The figure shows three views and two pictorial views of one solid part (mm, origin at its lowest corner). Answer the questions. Coordinates: 2 decimals unless noted, no trailing zeros. Write each loop counter-clockwise with the first axis right and the second up, starting at its lowest first coordinate (ties: lowest second). Pieces come first, ordered by that corner, then holes. Notation, with made-up numbers: (0, 35) - (31, 35) arc R18 ccw to (31, 66) - close; hole circle Ø4 at (14, 69). An arc over 180 degrees is marked (long way). Use a Markdown table: item, result. Add a question column.
(1) The part is cut by section A-A, the plane y = 0.75. Give the vertices of the cut face in (x, z), then the cut area to 3 significant figures.
(2) Find the intervals of material crossed by line 1 (X direction, y = 2.7, z = 16) (1 decimal); line 2 (X direction, y = 1.9, z = 92); line 3 (Z direction, x = 8.5, y = 1.7) (1 decimal), in increasing order. Write a range as from..to.
(3) The part is cut by section C-C, the plane x = 92. Give the vertices of the cut face in (y, z).
(4) The part is cut by section B-B, the plane z = 27.5. Give the vertices of the cut face in (x, y).
(5) Given pin 1 Ø1.5 at (y, z) = (2, 25.5) entering from +X, flat-ended and moving along its own axis, determine where the tip first touches the part or whether it passes through.
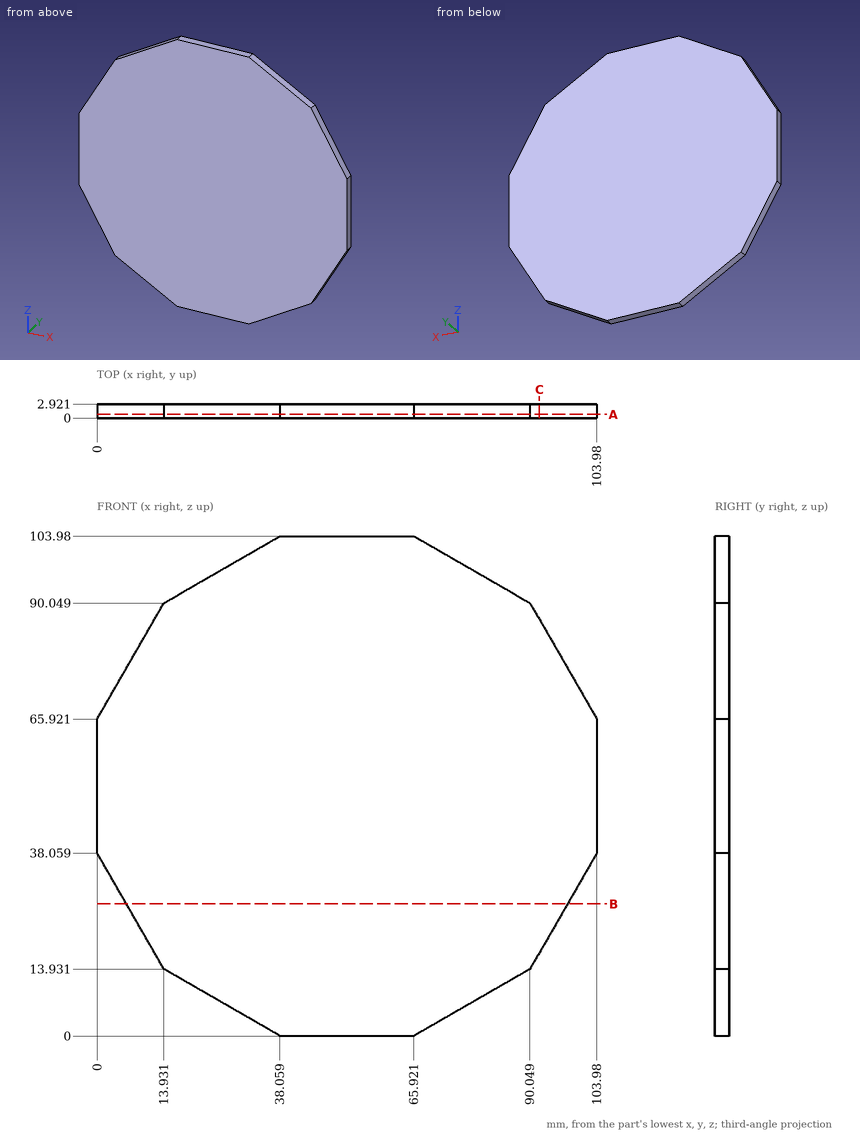
Model answer:
| question | item | result |
|---|---|---|
| 1 | outline | (0, 38.06) - (13.93, 13.93) - (38.06, 0) - (65.92, 0) - (90.05, 13.93) - (103.98, 38.06) - (103.98, 65.92) - (90.05, 90.05) - (65.92, 103.98) - (38.06, 103.98) - (13.93, 90.05) - (0, 65.92) - close |
| 1 | area | 8,690 mm^2 |
| 2 | line 1 | 12.7..91.2 |
| 2 | line 2 | 17.31..86.67 |
| 2 | line 3 | 23.3..80.6 |
| 3 | outline | (0, 17.31) - (2.92, 17.31) - (2.92, 86.67) - (0, 86.67) - close |
| 4 | outline | (6.1, 0) - (97.88, 0) - (97.88, 2.92) - (6.1, 2.92) - close |
| 5 | pin 1 | x = 97.16 |
